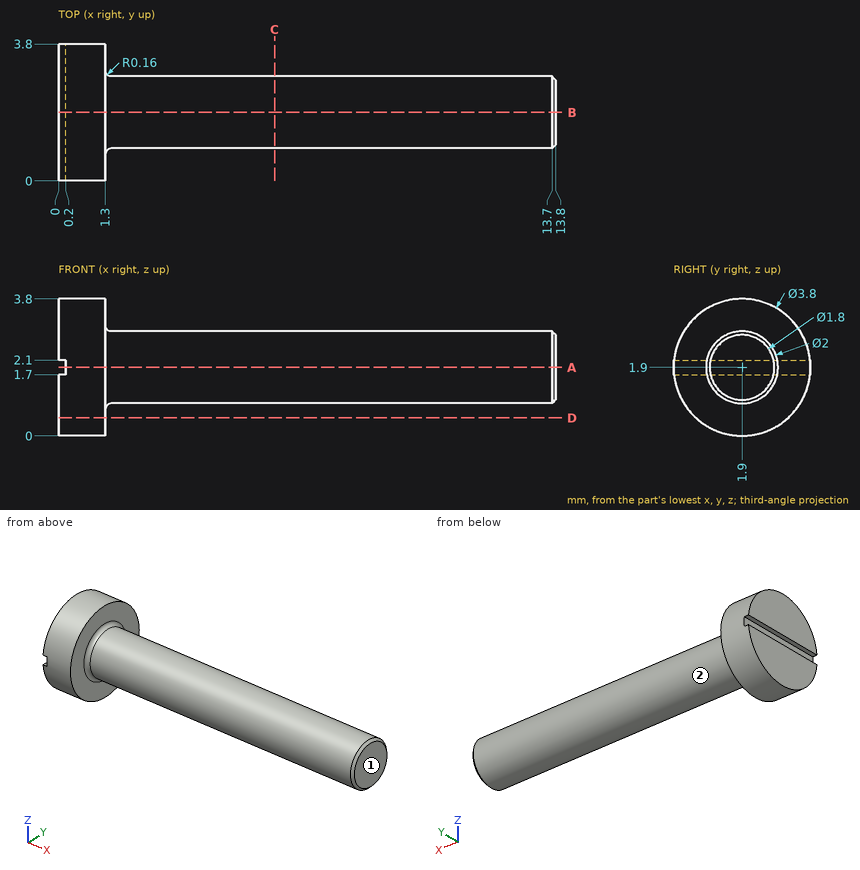
The figure shows three views and two pictorial views of one solid part (mm, origin at its lowest corner). Answer the questions. A direction names the side the tool comes from. Give positions to 0.01 mm unless a question says otherwise; leave off trailing zeros. Loops run counter-clockwise (first coordinate to the right, second up) from the corner with the lowest first, then second, coordinate; pieces in that order, holes last. Notation, with made-up numbers: (-5, 87.25) -> (10, 87.25) arc R25 ccw to (10, 102.25) -> close; hole circle Ø3 at (78.25, 70). An arc over 180 degrees is marked (long way). Put each result on its own line as item: value. Start each with the question number.
Item 1: Each of these flat-tipped pins is pushed along its axis until it touches: P1, Ø1.5, axis at x = 11, z = 2.5, coming from the +Y side; P2, Ø2, axis at x = 5.5, y = 2, coming from the +Z side; P3, Ø1, axis at x = 6.5, z = 1, coming from the -Y side. Where does it stop, or does it pass through?
Item 2: The part is cut by section A-A (z = 1.9). Give the vertices of the cut face in (x, y).
Item 3: Find the intervals of material crossed by L1, parallel to X at y = 0.35, z = 2.75; L2, parallel to Y at x = 1.25, z = 3.45; L3, parallel to Y at x = 8, z = 2.6, in increasing order. Write a range as [from, to].
Item 4: The part is cut by section C-C (x = 6). Give the vertices of the cut face in (y, z).
Item 5: The part is cut by section D-D (z = 0.5). Give the vertices of the cut face in (x, y), then the cut area to 3 significant figures.
Item 6: The part is cut by section B-B (y = 1.9). Give the vertices of the cut face in (x, z), then the cut area to 3 significant figures.
Item 7: Which of the six approach directions +Z, -Z, +X, -X, +Y, -Y give full straight-line access (tool end or side, diameter ignored) to the marked faces 1 and 2?
Answers below:
1. P1: y = 2.9
1. P2: z = 2.9
1. P3: y = 0.98
2. outline: (0.2, 0) -> (1.3, 0) -> (1.3, 0.74) arc R0.16 cw to (1.46, 0.9) -> (13.7, 0.9) -> (13.8, 1) -> (13.8, 2.8) -> (13.7, 2.9) -> (1.46, 2.9) arc R0.16 cw to (1.3, 3.06) -> (1.3, 3.8) -> (0.2, 3.8) -> close
3. L1: [0, 1.3]
3. L2: [0.8, 3]
3. L3: [1.19, 2.61]
4. outline: circle Ø2 at (1.9, 1.9)
5. outline: (0, 0.62) -> (1.3, 0.62) -> (1.3, 3.18) -> (0, 3.18) -> close
5. area: 3.34 mm2
6. outline: (0, 0) -> (1.3, 0) -> (1.3, 0.74) arc R0.16 cw to (1.46, 0.9) -> (13.7, 0.9) -> (13.8, 1) -> (13.8, 2.8) -> (13.7, 2.9) -> (1.46, 2.9) arc R0.16 cw to (1.3, 3.06) -> (1.3, 3.8) -> (0, 3.8) -> (0, 2.1) -> (0.2, 2.1) -> (0.2, 1.7) -> (0, 1.7) -> close
6. area: 29.9 mm2
7. face 1: +Z, -Z, +X, +Y, -Y
7. face 2: +X
